Could you check a few things on this drawing? It's one solid part, dimensions in mm from its lowest x, y, z. Coordinates: 2 decimals unless noted, no trailing zeros. Order: outer loops, then holes, each group sorted by start corner. A loop starts at its lowest first (then second) coordinate and runs counter-clockwise, first axis right, second up.
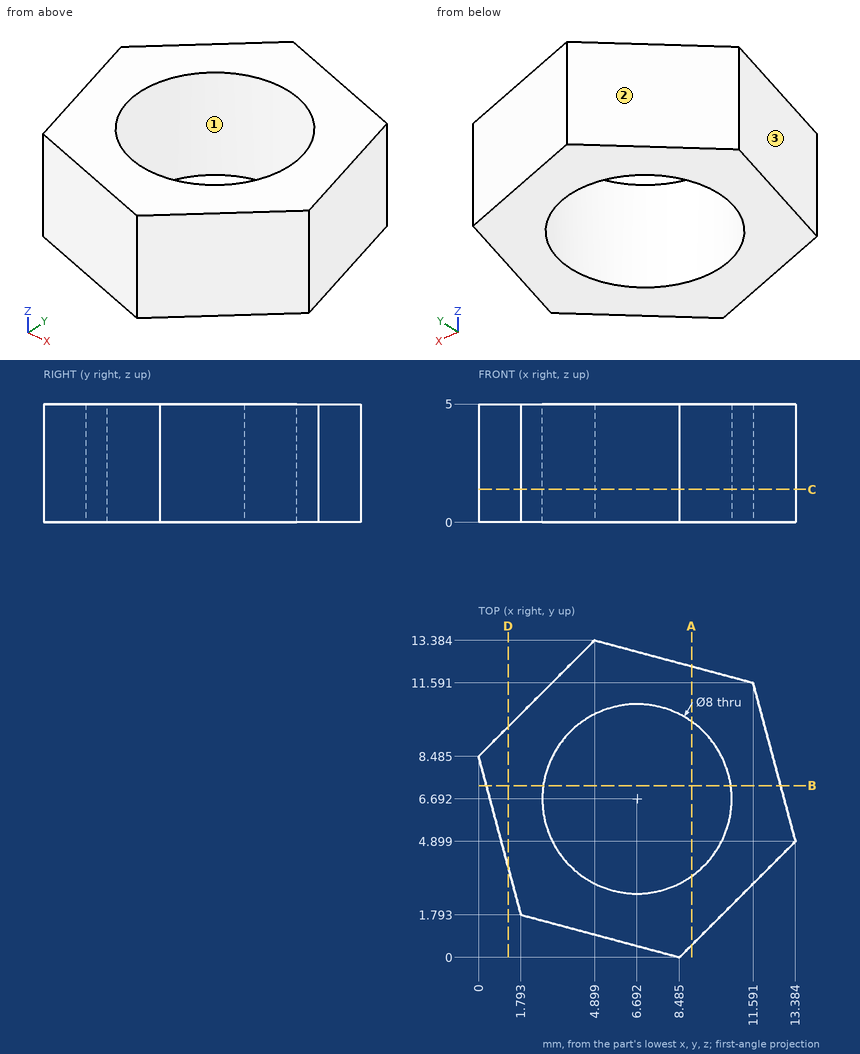
Q1. Will these pins go through, and if not, where does the flat tip stop? pin 1 (2 mm diameter, centred on y = 3.5, z = 3, fed in from -X); pin 2 (3 mm diameter, centred on x = 4.5, z = 4, fed in from -Y); pin 3 (7 mm diameter, centred on x = 6.69, y = 6.69, fed in from -Z); pin 4 (1.5 mm diameter, centred on x = 10, z = 1, fed in from -Y) (1 decimal).
Q2. If we section it at B-B on y = 7.25: Write out the boundary of the cut face in (x, z) (1 decimal), then the cut area to 3 significant figures.
Q3. We'd pull the mould along Y, two halves only. Please class the marked faces 1, 2 and 3: pulls with the +Y half, pulls with the -Y half, needs draft (parallel to the pull), parting line crosses it, or undercut.
Q4. I need wall thicknesses on L1, parallel to X at y = 9.25, z = 4.3 (1 decimal); L2, parallel to Y at x = 6, z = 2.75 (1 decimal); L3, parallel to X at y = 7.5, z = 3.55 (1 decimal). Which ranges of each line are inside material? Lowest first, please.
Q5. If we section it at D-D on x = 1.25: Write out the boundary of the cut face in (y, z) (1 decimal), then the cut area to 3 significant figures.
Q6. If we section it at C-C on z = 1.4: Write out the boundary of the cut face in (x, y) (1 decimal).
Q7. If we section it at A-A on x = 9: Write out the boundary of the cut face in (y, z) (1 decimal), then the cut area to 3 significant figures.
Reply:
1. pin 1: stops at x = 1.07
1. pin 2: stops at y = 0.67
1. pin 3: passes through
1. pin 4: stops at y = 0.8
2. outline: (0.3, 0) - (2.7, 0) - (2.7, 5) - (0.3, 5) - close; (10.7, 0) - (12.8, 0) - (12.8, 5) - (10.7, 5) - close
2. area: 22.5 mm2
3. face 1: undercut
3. face 2: pulls with the +Y half
3. face 3: pulls with the -Y half
4. L1: x = 0.8 to 3.6, 9.8 to 12.2
4. L2: y = 0.7 to 2.8, 10.6 to 13.1
4. L3: x = 0.3 to 2.8, 10.6 to 12.7
5. outline: (3.8, 0) - (9.7, 0) - (9.7, 5) - (3.8, 5) - close
5. area: 29.6 mm2
6. outline: (0, 8.5) - (1.8, 1.8) - (8.5, 0) - (13.4, 4.9) - (11.6, 11.6) - (4.9, 13.4) - close; hole circle Ø8 at (6.7, 6.7)
7. outline: (0.5, 0) - (3.4, 0) - (3.4, 5) - (0.5, 5) - close; (10, 0) - (12.3, 0) - (12.3, 5) - (10, 5) - close
7. area: 26.2 mm2
